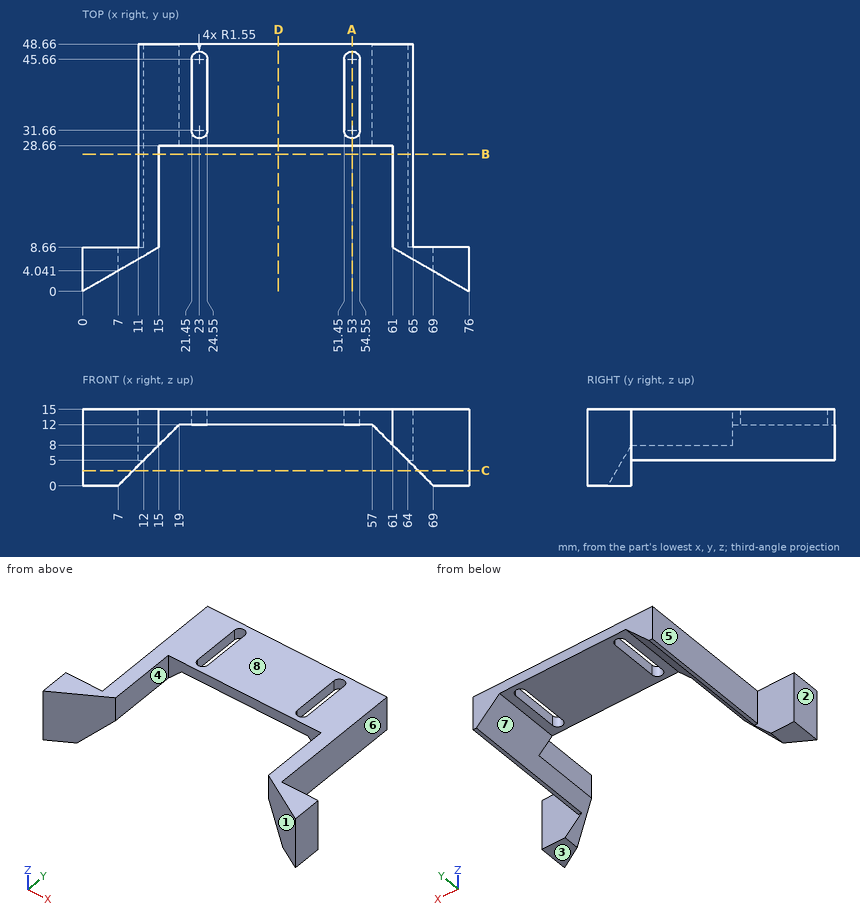
Input: dimensioned drawing with shaded views. Units: mm. Origin: part minimum x, y, z. A direction names the side the tool comes from. Round coordinates to 2 decimals unless told otherwise and drop trailing zeros. Order: outer loops, then holes, each group sorted by start corner. A loop starts at its lowest first (then second) coordinate and runs counter-clockwise, first axis right, second up. Notation, with made-up numbers: (-24, 33.25) - (26, 33.25) arc R32 cw to (26, 63.25) - close; hole circle Ø9 at (-31, 83). An arc over 180 degrees is marked (long way). Write item = value, one per line. Start each with the question number.
Q1. Cut plane D-D on x = 38.5. Return the cut outline in (y, z).
Q2. Cut plane A-A on x = 53. Return the cut outline in (y, z).
Q3. Access query for the marked faces 4, 5, 6, 7 and 8. Directions: +Z, -Z, +X, -X, +Y, -Y. A direction counts if a zero-diameter tool reaches every point of the face in a straight line with its end or side. Return the directions, or none.
Q4. Cut plane B-B on y = 27. Return the cut outline in (x, z).
Q5. Pin query (flat end, axial travel): pin 1 (1.5 mm diameter, centred on y = 38.5, z = 13, fed in from +X); pin 2 (1.1 mm diameter, centred on x = 11.5, y = 20, fed in from -Z); pin 3 (5.5 mm diameter, centred on y = 14, z = 10, fed in from -X). Return the tip coordinate at first contact, or that it passes through.
Q6. Pull-direction query (X, two-part tool) for the marked faces 1, 2 and 3; classes: +X half, -X half, draft (parallel to the pull), parting line (faces both ways), or undercut.
Q7. Cut plane C-C on z = 3. Return the cut outline in (x, y).
Q8. Ray query, line 1 (Z direction, x = 27, y = 37); line 2 (X direction, y = 2, z = 2) (1 decimal); line 3 (X direction, y = 23, z = 10.5). Return the intervals inside material, ascending. Write a range as from..to.
Outcome:
q1.outline = (28.66, 12) - (48.66, 12) - (48.66, 15) - (28.66, 15) - close
q2.outline = (28.66, 12) - (30.11, 12) - (30.11, 15) - (28.66, 15) - close; (47.21, 12) - (48.66, 12) - (48.66, 15) - (47.21, 15) - close
q3.face_4 = +Z, -Z, -Y
q3.face_5 = +Z, -Z, -X, +Y
q3.face_6 = +Z, -Z, +X, +Y
q3.face_7 = -Z, +Y, -Y
q3.face_8 = +Z, +X, -X, +Y, -Y
q4.outline = (11, 5) - (12, 5) - (15, 8) - (15, 15) - (11, 15) - close; (61, 8) - (64, 5) - (65, 5) - (65, 15) - (61, 15) - close
q5.pin_1 = 65
q5.pin_2 = 5
q5.pin_3 = 11
q6.face_1 = undercut
q6.face_2 = -X half
q6.face_3 = draft
q7.outline = (0, 0) - (10, 5.77) - (10, 8.66) - (0, 8.66) - close; (66, 5.77) - (76, 0) - (76, 8.66) - (66, 8.66) - close
q8.line_1 = 12..15
q8.line_2 = 0..3.5, 72.5..76
q8.line_3 = 11..15, 61..65
